The model under review builds one solid part; all positions refer to its coordinate system, in mm. A direction names the side the tool comes from. Coordinates: 2 decimals unless noted, no trailing zeros. Order: outer loops, then holes, each group sorted by start corner. A loop starts at its lowest first (then second) coordinate and runs counter-clockwise, first axis right, second up. Notation, with made-up numbers: (87, -8) - (104, -8) arc R32 cw to (104, 29) - close; hole circle Ø11 at (78.25, -18). An arc over 180 degrees is marked (long way). Answer in a Markdown table with one row per item.
```python
from build123d import *

# Parameters (mm, degrees)
SKETCH_1_W              = 350
SKETCH_1_H              = 130
EXTRUDE_1_DEPTH         = 3
SKETCH_2_R              = 2.1
CUT_EXTRUDE_1_DEPTH     = 191.417961338
SKETCH_3_R              = 32
SKETCH_3_R_2            = 38
CUT_EXTRUDE_3_DEPTH     = 10
SKETCH_4_W              = 40
SKETCH_4_H              = 15
CUT_EXTRUDE_4_DEPTH     = 191.417961338
HOLE_WIZARD_4_2_4_2_1_D = 4.2
HOLE_WIZARD_3_2_3_2_2_D = 3.2
CUT_EXTRUDE_5_DEPTH     = 191.417961338
CUT_EXTRUDE_6_DEPTH     = 191.417961338
FILLET_1_R              = 4
CUT_EXTRUDE_7_DEPTH     = 191.417961338
FILLET_2_R              = 2
FILLET_2_OF_MIRROR_4_R  = 2
HOLE_WIZARD_3_2_3_2_3_D = 3.2


with BuildPart() as part:
    # 草图1 → 凸台-拉伸1 (new body)
    with BuildSketch(Plane.XY):
        with Locations((0, 10)):
            Rectangle(SKETCH_1_W, SKETCH_1_H)
    extrude(amount=EXTRUDE_1_DEPTH)

    # 草图2 → 切除-拉伸1 (cut, through all)
    with BuildSketch(Plane(origin=(0, 0, 0), x_dir=(-1, 0, 0), z_dir=(0, 0, -1))):
        with Locations((-100, 42)):
            Circle(SKETCH_2_R)
        with Locations((-70.30151519, 29.69848481)):
            Circle(SKETCH_2_R)
        with Locations((-58, 0)):
            Circle(SKETCH_2_R)
        with Locations((-70.30151519, -29.69848481)):
            Circle(SKETCH_2_R)
        with Locations((-100, -42)):
            Circle(SKETCH_2_R)
        with Locations((-129.69848481, -29.69848481)):
            Circle(SKETCH_2_R)
        with Locations((-142, 0)):
            Circle(SKETCH_2_R)
        with Locations((-129.69848481, 29.69848481)):
            Circle(SKETCH_2_R)
        with Locations(Location((129.69848481, 29.69848481, 0), (0, 0, 180))):
            Circle(SKETCH_2_R)
        with Locations(Location((142, 0, 0), (0, 0, 180))):
            Circle(SKETCH_2_R)
        with Locations(Location((129.69848481, -29.69848481, 0), (0, 0, 180))):
            Circle(SKETCH_2_R)
        with Locations(Location((100, -42, 0), (0, 0, 180))):
            Circle(SKETCH_2_R)
        with Locations(Location((70.30151519, -29.69848481, 0), (0, 0, 180))):
            Circle(SKETCH_2_R)
        with Locations(Location((58, 0, 0), (0, 0, 180))):
            Circle(SKETCH_2_R)
        with Locations(Location((70.30151519, 29.69848481, 0), (0, 0, 180))):
            Circle(SKETCH_2_R)
        with Locations(Location((100, 42, 0), (0, 0, 180))):
            Circle(SKETCH_2_R)
    extrude(amount=-CUT_EXTRUDE_1_DEPTH, mode=Mode.SUBTRACT)

    # 草图3 → 切除-拉伸3 (cut)
    with BuildSketch(Plane(origin=(0, 0, 0), x_dir=(-1, 0, 0), z_dir=(0, 0, -1))):
        with Locations((-100, 0)):
            Circle(SKETCH_3_R)
        with Locations((100, 0)):
            Circle(SKETCH_3_R_2)
    extrude(amount=-CUT_EXTRUDE_3_DEPTH, mode=Mode.SUBTRACT)

    # 草图4 → 切除-拉伸4 (cut, through all)
    with BuildSketch(Plane(origin=(0, 0, 0), x_dir=(-1, 0, 0), z_dir=(0, 0, -1))):
        with Locations((100, 37.5)):
            Rectangle(SKETCH_4_W, SKETCH_4_H)
    extrude(amount=-CUT_EXTRUDE_4_DEPTH, mode=Mode.SUBTRACT)

    # Ø4.2 (4.2) 直径孔1 (through all)
    with Locations(Plane(origin=(-30, 65, 3), x_dir=(1, 0, 0), z_dir=(0, 0, 1))):
        with Locations((0, 0), (-40, 0), (-85, 0), (-105, 0)):
            hole_wizard_4_2_4_2_1 = Hole(HOLE_WIZARD_4_2_4_2_1_D / 2)

    # 镜向1: Ø4.2 (4.2) 直径孔1 across plane
    add(hole_wizard_4_2_4_2_1.mirror(Plane(origin=(0, 0, 0), x_dir=(0, 0, 1), z_dir=(1, 0, 0))), mode=Mode.SUBTRACT)

    # Ø3.2 (3.2) 直径孔2 (through all)
    with Locations(Plane(origin=(-172, 25, 3), x_dir=(1, 0, 0), z_dir=(0, 0, 1))):
        with Locations((0, 0), (0, -20)):
            hole_wizard_3_2_3_2_2 = Hole(HOLE_WIZARD_3_2_3_2_2_D / 2)

    # 镜向3: Ø3.2 (3.2) 直径孔2 across plane
    add(hole_wizard_3_2_3_2_2.mirror(Plane(origin=(0, 0, 0), x_dir=(0, 0, 1), z_dir=(1, 0, 0))), mode=Mode.SUBTRACT)

    # 草图12 → 切除-拉伸5 (cut, through all)
    with BuildSketch(Plane.XY.offset(3)):
        with BuildLine():
            Line((-175, -55), (-100, -55))
            ThreePointArc((-100, -55), (-120.310096012, -51.112620751), (-137.749172176, -40))
            Line((-137.749172176, -40), (-175, -40))
            Line((-175, -40), (-175, -55))
        make_face()
        with BuildLine():
            Line((175, -55), (175, -40))
            Line((175, -40), (137.749172176, -40))
            ThreePointArc((137.749172176, -40), (120.310096012, -51.112620751), (100, -55))
            Line((100, -55), (175, -55))
        make_face()
    extrude(amount=-CUT_EXTRUDE_5_DEPTH, mode=Mode.SUBTRACT)

    # 草图14 → 切除-拉伸6 (cut, through all)
    with BuildSketch(Plane.XY.offset(3)):
        with BuildLine():
            Line((-62.250827824, -40), (62.250827824, -40))
            ThreePointArc((62.250827824, -40), (79.689903988, -51.112620751), (100, -55))
            Line((100, -55), (-100, -55))
            ThreePointArc((-100, -55), (-79.689903988, -51.112620751), (-62.250827824, -40))
        make_face()
    extrude(amount=-CUT_EXTRUDE_6_DEPTH, mode=Mode.SUBTRACT)

    # 圆角1
    fillet_1_edges = [part.edges().sort_by_distance(p)[0] for p in [
        (-120, 45, 1.5),
        (-80, 45, 1.5),
        (-120, 32.310988843, 1.5),
        (-80, 32.310988843, 1.5),
    ]]
    fillet(fillet_1_edges, radius=FILLET_1_R)

    # 草图16 → 切除-拉伸7 (cut, through all)
    with BuildSketch(Plane.XY.offset(3)):
        with BuildLine():
            Line((76.020842383, 55), (5, 55))
            Line((5, 55), (51.266028276, 35))
            ThreePointArc((51.266028276, 35), (62.293239404, 46.671192457), (76.020842383, 55))
        make_face()
        with BuildLine():
            Line((46.091915187, 26.342330797), (32.537213763, 32.201792665))
            Line((32.537213763, 32.201792665), (20.206140943, 3.676304477))
            Line((20.206140943, 3.676304477), (40.206140943, -4.969347957))
            ThreePointArc((40.206140943, -4.969347957), (41.032735212, 11.084298962), (46.091915187, 26.342330797))
        make_face()
        Polygon((5, 44.105651626), (5, -6.298171369), (23.358142509, 36.169745652), align=None)
        with BuildLine():
            Line((42.404028194, -16.813804795), (16.238187957, -5.502766777))
            Line((16.238187957, -5.502766777), (7.809872863, -25))
            Line((7.809872863, -25), (45.456439427, -25))
            ThreePointArc((45.456439427, -25), (43.781034085, -20.962534948), (42.404028194, -16.813804795))
        make_face()
    cut_extrude_7 = extrude(amount=-CUT_EXTRUDE_7_DEPTH, mode=Mode.SUBTRACT)

    # 圆角2
    fillet_2_edges = [part.edges().sort_by_distance(p)[0] for p in [
        (42.404028194, -16.813804795, 1.5),
        (45.456439427, -25, 1.5),
        (7.809872863, -25, 1.5),
        (16.238187957, -5.502766777, 1.5),
        (20.206140943, 3.676304477, 1.5),
        (32.537213763, 32.201792665, 1.5),
        (46.091915187, 26.342330797, 1.5),
        (40.206140943, -4.969347957, 1.5),
        (5, 44.105651626, 1.5),
        (23.358142509, 36.169745652, 1.5),
        (5, -6.298171369, 1.5),
        (51.266028276, 35, 1.5),
        (5, 55, 1.5),
        (76.020842383, 55, 1.5),
    ]]
    fillet(fillet_2_edges, radius=FILLET_2_R)

    # 镜向4: 切除-拉伸7 across plane
    add(cut_extrude_7.mirror(Plane(origin=(0, 0, 0), x_dir=(0, 0, 1), z_dir=(1, 0, 0))), mode=Mode.SUBTRACT)

    # 圆角2 of 镜向4
    fillet_2_of_mirror_4_edges = [part.edges().sort_by_distance(p)[0] for p in [
        (-42.404028194, -16.813804795, 1.5),
        (-45.456439427, -25, 1.5),
        (-7.809872863, -25, 1.5),
        (-16.238187957, -5.502766777, 1.5),
        (-20.206140943, 3.676304477, 1.5),
        (-32.537213763, 32.201792665, 1.5),
        (-46.091915187, 26.342330797, 1.5),
        (-40.206140943, -4.969347957, 1.5),
        (-5, 44.105651626, 1.5),
        (-23.358142509, 36.169745652, 1.5),
        (-5, -6.298171369, 1.5),
        (-51.266028276, 35, 1.5),
        (-5, 55, 1.5),
        (-76.020842383, 55, 1.5),
    ]]
    fillet(fillet_2_of_mirror_4_edges, radius=FILLET_2_OF_MIRROR_4_R)

    # Ø3.2 (3.2) 直径孔3 (through all)
    with Locations(Plane(origin=(18, -37, 3), x_dir=(1, 0, 0), z_dir=(0, 0, 1))):
        with Locations((0, 0), (20, 0)):
            hole_wizard_3_2_3_2_3 = Hole(HOLE_WIZARD_3_2_3_2_3_D / 2)

    # 镜向5: Ø3.2 (3.2) 直径孔3 across plane
    add(hole_wizard_3_2_3_2_3.mirror(Plane(origin=(0, 0, 0), x_dir=(0, 0, 1), z_dir=(1, 0, 0))), mode=Mode.SUBTRACT)


solid = part.part
```
Item 1: We need section A-A, the plane x = 109. Write out the cut boundary in (y, z).
Check values:
| item | result |
|---|---|
| outline | (-54.26, 0) - (-30.71, 0) - (-30.71, 3) - (-54.26, 3) - close; (30.71, 0) - (75, 0) - (75, 3) - (30.71, 3) - close |
Item 2: To check wall thickness, follow line 1 (Y direction, x = -172, z = 2.05); line 2 (Y direction, x = -101, z = 2.3); line 3 (Y direction, x = -70, z = 1.1). State the ranges of each line that lie inside material, in increasing order. Write a range as from..to.
Check values:
| item | result |
|---|---|
| line 1 | -40..3.4, 6.6..23.4, 26.6..75 |
| line 2 | -54.99..-43.85, -40.15..-37.99, 45..75 |
| line 3 | -46.1..-31.78, -27.62..-23.32, 23.32..27.62, 31.78..62.9, 67.1..75 |
Item 3: We need section B-B, the plane y = 19. Write out the cut boundary in (x, z).
Check values:
| item | result |
|---|---|
| outline | (-175, 0) - (-132.91, 0) - (-132.91, 3) - (-175, 3) - close; (-67.09, 0) - (-43.09, 0) - (-43.09, 3) - (-67.09, 3) - close; (-26.83, 0) - (-15.94, 0) - (-15.94, 3) - (-26.83, 3) - close; (-5, 0) - (5, 0) - (5, 3) - (-5, 3) - close; (15.94, 0) - (26.83, 0) - (26.83, 3) - (15.94, 3) - close; (43.09, 0) - (74.25, 0) - (74.25, 3) - (43.09, 3) - close; (125.75, 0) - (175, 0) - (175, 3) - (125.75, 3) - close |
Item 4: Clearance check with flat-ended pins moving along their axes: pin 1 Ø3.5 at (x, y) = (-135, 65) entering from +Z; pin 2 Ø0.9 at (x, z) = (-107, 1) entering from -Y. State where each tip first meets the part, or that it passes through.
Check values:
| item | result |
|---|---|
| pin 1 | through |
| pin 2 | y = -54.61 |
Item 5: Tool access review of faces 1 (the face through (-2, 25, 0)), 2 (the face through (29.976, -11.441, 1.521)): name each direction out of +Z, -Z, +X, -X, +Y, -Y from which nothing blocks a thin tool from reaching the whole face with its end or side.
Check values:
| item | result |
|---|---|
| face 1 | -Z, +X, -X, +Y, -Y |
| face 2 | +Z, -Z |
Item 6: Mouldability with a two-part tool opening along X and no side actions: class faces 3 (the face through (31.6, 43.5, 1.5)), 4 (the face through (-2, 25, 3)) as +X half, -X half, draft (parallel to the pull), parting line (faces both ways), or undercut.
Check values:
| item | result |
|---|---|
| face 3 | undercut |
| face 4 | draft |
Item 7: We need section C-C, the plane z = 1.6. State how many separate pieces and enclosed holes the cut face has, then the cut area to 3 significant figures.
Check values:
| item | result |
|---|---|
| separate pieces | 1 |
| enclosed holes | 41 |
| area | 29,200 mm^2 |
